```python
from build123d import *

# Parameters (mm, degrees)
CROQUIS1_R                 = 10.5
CROQUIS1_R_2               = 4
SALIENTE_EXTRUIR1_DEPTH    = 15
CORTAR_EXTRUIR1_DEPTH      = 15
CORTAR_EXTRUIR1_DEPTH_BACK = 15
CROQUIS2_R                 = 1
CORTAR_EXTRUIR2_DEPTH      = 15
CORTAR_EXTRUIR2_DEPTH_BACK = 15
CROQUIS3_R                 = 1.002014624


with BuildPart() as part:
    # Croquis1 → Saliente-Extruir1 (new body)
    with BuildSketch(Plane(origin=(0, 0, 0), x_dir=(1, 0, 0), z_dir=(0, 1, 0))):
        with Locations(Location((0, 0, 0), (0, 0, 270))):
            Circle(CROQUIS1_R)
        with Locations(Location((0, 0, 0), (0, 0, 270))):
            Circle(CROQUIS1_R_2, mode=Mode.SUBTRACT)
    extrude(amount=SALIENTE_EXTRUIR1_DEPTH)

    # Croquis2 → Cortar-Extruir1 (cut, two sides: drawn at the far end of the back side and taken through both)
    with BuildSketch(Plane.XY.offset(-CORTAR_EXTRUIR1_DEPTH_BACK)):
        with Locations(Location((0, 12.5, 0), (0, 0, 180))):
            Circle(CROQUIS2_R)
    extrude(amount=CORTAR_EXTRUIR1_DEPTH + CORTAR_EXTRUIR1_DEPTH_BACK, mode=Mode.SUBTRACT)

    # Croquis3 → Cortar-Extruir2 (cut, two sides: drawn at the far end of the back side and taken through both)
    with BuildSketch(Plane(origin=(0, 0, 0), x_dir=(0, 0, -1), z_dir=(1, 0, 0)).offset(-CORTAR_EXTRUIR2_DEPTH_BACK)):
        with Locations(Location((0.063508327, 12.5, 0), (0, 0, 180))):
            Circle(CROQUIS3_R)
    extrude(amount=CORTAR_EXTRUIR2_DEPTH + CORTAR_EXTRUIR2_DEPTH_BACK, mode=Mode.SUBTRACT)


solid = part.part
```
Verification items for the finished model (mm, model axes). Give positions to 0.01 mm unless a question says otherwise; leave off trailing zeros. Order: outer loops, then holes, each group sorted by start corner. A loop starts at its lowest first (then second) coordinate and runs counter-clockwise, first axis right, second up. Notation, with made-up numbers: M 85.5,34 L 100.5,34 A26 ccw 100.5,71 Z; hole C 31,-16 d5. An arc over 180 degrees is marked long. Answer in a Markdown table with one row per item. Add a question column.
Item 1: Mould release check, pull along Y, two halves, no side actions. Record for faces 1 (the flat face through (0, 0, 5)), 2 (the cylindrical face through (-0.46, 13.39, 7.14)), 3 (the flat face through (0, 15, 5)), 4 (the cylindrical face through (-0.46, 13.39, -7.23)): released by +Y, released by -Y, zero draft, split by the parting line, or undercut.
Item 2: Gauge pin test, flat ends, axial feed: pin 1 (4 mm diameter, centred on x = 1, y = 7.5, fed in from -Z); pin 2 (2 mm diameter, centred on y = 8.5, z = 3, fed in from +X); pin 3 (6 mm diameter, centred on x = 6.5, y = 11, fed in from +Z); pin 4 (6 mm diameter, centred on x = 8, y = 13, fed in from +Z). Record the tip position at first contact, or that the pin passes through.
Item 3: Scan lines: probe 1 along Z at (x, y) = (0, 9.5); probe 2 along Y at (x, z) = (-4.5, 0). Record each from-to range of solid material in increasing order. Write a range as from..to.
Item 4: Section check D-D, the plane x = -7.25. Enter the section's corners in (y, z).
Item 5: Section check C-C, the plane y = 4. Enter the section's corners in (x, z), and give its area (3 significant figures).
Item 6: Section check B-B, the plane z = 0. Enter the section's corners in (x, y).
Item 7: Section check A-A, the plane x = 0. Enter the section's corners in (y, z), and give its area (3 significant figures).
Filled sheet:
| question | item | result |
|---|---|---|
| 1 | face 1 | released by -Y |
| 1 | face 2 | undercut |
| 1 | face 3 | released by +Y |
| 1 | face 4 | undercut |
| 2 | pin 1 | stops at z = -10.5 |
| 2 | pin 2 | stops at x = 10.31 |
| 2 | pin 3 | stops at z = 9.9 |
| 2 | pin 4 | stops at z = 9.23 |
| 3 | probe 1 | z = -10.5..-4, 4..10.5 |
| 3 | probe 2 | y = 0..11.5, 13.5..15 |
| 4 | outline | M 0,-7.6 L 15,-7.6 L 15,7.6 L 0,7.6 Z; hole C 12.5,-0.06 d2 |
| 5 | outline | C 0,0 d21; hole C 0,0 d8 |
| 5 | area | 296 mm^2 |
| 6 | outline | M -10.5,0 L -4,0 L -4,11.5 L -10.5,11.5 Z; M -10.5,13.5 L -4,13.5 L -4,15 L -10.5,15 Z; M 4,0 L 10.5,0 L 10.5,11.5 L 4,11.5 Z; M 4,13.5 L 10.5,13.5 L 10.5,15 L 4,15 Z |
| 7 | outline | M 0,-10.5 L 11.5,-10.5 L 11.5,-4 L 0,-4 Z; M 0,4 L 11.5,4 L 11.5,10.5 L 0,10.5 Z; M 13.5,-10.5 L 15,-10.5 L 15,-4 L 13.5,-4 Z; M 13.5,4 L 15,4 L 15,10.5 L 13.5,10.5 Z |
| 7 | area | 169 mm^2 |
